Source: CAD feature listing. Evaluate the final solid. Frame: model axes, mm. A direction names the side the tool comes from. Give positions to 0.01 mm unless a question says otherwise; leave off trailing zeros. Loops run counter-clockwise (first coordinate to the right, second up) from the corner with the lowest first, then second, coordinate; pieces in that order, holes last.
```python
from build123d import *

# Parameters (mm, degrees)
F0_W     = 56.8
F0_H     = 54
F1_DEPTH = 1.8
F2_W     = 23.4
F2_H     = 12.8
F2_R     = 0.85
F3_DEPTH = 1.801
F4_R     = 1.5
F5_R     = 1.75
F5_R_2   = 0.85
F6_DEPTH = 1.4
F7_R     = 4.5
F8_DEPTH = 0.2


# Not quite as in the source:
# - a pattern or mirror of a feature is missing from the dataset's text; its kind, count and spacing are read off the source's solid


with BuildPart() as f1:
    # F0 (on Top) → F1 (new body)
    with BuildSketch(Plane.XY):
        Rectangle(F0_W, F0_H)
    extrude(amount=F1_DEPTH)

    # F2 (on face) → F3 (cut, through all)
    with BuildSketch(Plane.XY.offset(1.8)):
        with Locations((6.7, 10.6)):
            Rectangle(F2_W, F2_H)
        with Locations((-7.05, 10.6)):
            Circle(F2_R)
        with Locations((20.45, 10.6)):
            Circle(F2_R)
    f3 = extrude(amount=-F3_DEPTH, mode=Mode.SUBTRACT)

    # F3_copies: F3 across plane
    add(f3.mirror(Plane(origin=(0, 0, 0), x_dir=(0, 0, -1), z_dir=(0, -1, 0))), mode=Mode.SUBTRACT)

    # F4
    f4_edges = [f1.edges().sort_by_distance(p)[0] for p in [
        (28.4, 27, 0.9),
        (28.4, -27, 0.9),
        (-28.4, -27, 0.9),
        (-28.4, 27, 0.9),
    ]]
    fillet(f4_edges, radius=F4_R)

    # F5 (on face) → F6 (join)
    with BuildSketch(Plane(origin=(0, 0, 0), x_dir=(1, 0, 0), z_dir=(0, 0, -1))):
        with BuildLine():
            Line((-28.4, 25.5), (-28.4, -25.5))
            ThreePointArc((-28.4, -25.5), (-27.9606601718, -26.5606601718), (-26.9, -27))
            Line((-26.9, -27), (26.9, -27))
            ThreePointArc((26.9, -27), (27.9606601718, -26.5606601718), (28.4, -25.5))
            Line((28.4, -25.5), (28.4, 25.5))
            ThreePointArc((28.4, 25.5), (27.9606601718, 26.5606601718), (26.9, 27))
            Line((26.9, 27), (-26.9, 27))
            ThreePointArc((-26.9, 27), (-27.9606601718, 26.5606601718), (-28.4, 25.5))
        make_face()
        with BuildLine():
            Line((26.8, -2), (26.8, -24.4))
            ThreePointArc((26.8, -24.4), (26.5071067812, -25.1071067812), (25.8, -25.4))
            Line((25.8, -25.4), (-25.8, -25.4))
            ThreePointArc((-25.8, -25.4), (-26.5071067812, -25.1071067812), (-26.8, -24.4))
            Line((-26.8, -24.4), (-26.8, -2))
            Line((-26.8, -2), (-26.8, 2))
            Line((-26.8, 2), (-26.8, 24.4))
            ThreePointArc((-26.8, 24.4), (-26.5071067812, 25.1071067812), (-25.8, 25.4))
            Line((-25.8, 25.4), (25.8, 25.4))
            ThreePointArc((25.8, 25.4), (26.5071067812, 25.1071067812), (26.8, 24.4))
            Line((26.8, 24.4), (26.8, 2))
            Line((26.8, 2), (26.8, -2))
        make_face(mode=Mode.SUBTRACT)
        with Locations((-7.05, 10.6)):
            Circle(F5_R)
        with Locations((-7.05, 10.6)):
            Circle(F5_R_2, mode=Mode.SUBTRACT)
        with Locations((-7.05, -10.6)):
            Circle(F5_R)
        with Locations((-7.05, -10.6)):
            Circle(F5_R_2, mode=Mode.SUBTRACT)
        with Locations((20.45, 10.6)):
            Circle(F5_R)
        with Locations((20.45, 10.6)):
            Circle(F5_R_2, mode=Mode.SUBTRACT)
        with Locations((20.45, -10.6)):
            Circle(F5_R)
        with Locations((20.45, -10.6)):
            Circle(F5_R_2, mode=Mode.SUBTRACT)
        with BuildLine():
            ThreePointArc((25.6, -0.8), (26.4485281374, -1.1514718626), (26.8, -2))
            Line((26.8, -2), (26.8, 2))
            ThreePointArc((26.8, 2), (26.4485281374, 1.1514718626), (25.6, 0.8))
            Line((25.6, 0.8), (-25.6, 0.8))
            ThreePointArc((-25.6, 0.8), (-26.4485281374, 1.1514718626), (-26.8, 2))
            Line((-26.8, 2), (-26.8, -2))
            ThreePointArc((-26.8, -2), (-26.4485281374, -1.1514718626), (-25.6, -0.8))
            Line((-25.6, -0.8), (25.6, -0.8))
        make_face()
    extrude(amount=F6_DEPTH)

    # F7 (on face) → F8 (join)
    with BuildSketch(Plane.XY.offset(1.8)):
        with Locations((-26.9, 25.5)):
            Circle(F7_R)
        with Locations((-26.9, -25.5)):
            Circle(F7_R)
        with Locations((26.9, -25.5)):
            Circle(F7_R)
        with Locations((26.9, 25.5)):
            Circle(F7_R)
    extrude(amount=-F8_DEPTH)


solid = f1.part
```
(1) First-contact query: pin 1 (0.5 mm diameter, centred on x = 8, z = 1, fed in from -Y); pin 2 (1.4 mm diameter, centred on y = -12, z = 1, fed in from +X); pin 3 (0.9 mm diameter, centred on x = 1.5, z = 1, fed in from +Y). Flat tips, straight axial feed; report the tip coordinate or a pass-through.
A:
pin 1: stops at y = -27
pin 2: stops at x = 28.4
pin 3: stops at y = 27
(2) Ray query, line 1 along Y through (x, z) = (20.45, 1.1); line 2 along Y through (x, z) = (0, 1.05); line 3 along X through (y, z) = (-10.6, 0.8). Return the intervals inside material, ascending.
A:
line 1: y = -27 to -11.45, -9.75 to 9.75, 11.45 to 27
line 2: y = -27 to -17, -4.2 to 4.2, 17 to 27
line 3: x = -28.4 to -7.9, -6.2 to -5, 18.4 to 19.6, 21.3 to 28.4
(3) Section C-C, the plane z = 0.55. Return the cut outline in (x, y).
A:
outline: (-28.4, -25.5) arc R1.5 ccw to (-26.9, -27) - (26.9, -27) arc R1.5 ccw to (28.4, -25.5) - (28.4, 25.5) arc R1.5 ccw to (26.9, 27) - (-26.9, 27) arc R1.5 ccw to (-28.4, 25.5) - close; hole circle Ø1.7 at (-7.05, -10.6); hole circle Ø1.7 at (-7.05, 10.6); hole (-5, -17) - (18.4, -17) - (18.4, -4.2) - (-5, -4.2) - close; hole (-5, 4.2) - (18.4, 4.2) - (18.4, 17) - (-5, 17) - close; hole circle Ø1.7 at (20.45, -10.6); hole circle Ø1.7 at (20.45, 10.6)
(4) Section D-D, the plane y = -10.6. Return the cut outline in (x, z), then the cut area to 3 significant figures.
A:
outline: (-28.4, -1.4) - (-26.8, -1.4) - (-26.8, 0) - (-8.8, 0) - (-8.8, -1.4) - (-7.9, -1.4) - (-7.9, 1.8) - (-28.4, 1.8) - close; (-6.2, -1.4) - (-5.3, -1.4) - (-5.3, 0) - (-5, 0) - (-5, 1.8) - (-6.2, 1.8) - close; (18.4, 0) - (18.7, 0) - (18.7, -1.4) - (19.6, -1.4) - (19.6, 1.8) - (18.4, 1.8) - close; (21.3, -1.4) - (22.2, -1.4) - (22.2, 0) - (26.8, 0) - (26.8, -1.4) - (28.4, -1.4) - (28.4, 1.8) - (21.3, 1.8) - close
area: 63.5 mm2
(5) Section A-A, the plane x = 20.45. Return the cut outline in (y, z), then the cut area to 3 significant figures.
A:
outline: (-27, -1.4) - (-25.4, -1.4) - (-25.4, 0) - (-12.35, 0) - (-12.35, -1.4) - (-11.45, -1.4) - (-11.45, 1.8) - (-27, 1.8) - close; (-9.75, -1.4) - (-8.85, -1.4) - (-8.85, 0) - (-0.8, 0) - (-0.8, -1.4) - (0.8, -1.4) - (0.8, 0) - (8.85, 0) - (8.85, -1.4) - (9.75, -1.4) - (9.75, 1.8) - (-9.75, 1.8) - close; (11.45, -1.4) - (12.35, -1.4) - (12.35, 0) - (25.4, 0) - (25.4, -1.4) - (27, -1.4) - (27, 1.8) - (11.45, 1.8) - close
area: 103 mm2
(6) Section B-B, the plane y = 16. Return the cut outline in (x, z), then the cut area to 3 significant figures.
A:
outline: (-28.4, -1.4) - (-26.8, -1.4) - (-26.8, 0) - (-5, 0) - (-5, 1.8) - (-28.4, 1.8) - close; (18.4, 0) - (26.8, 0) - (26.8, -1.4) - (28.4, -1.4) - (28.4, 1.8) - (18.4, 1.8) - close
area: 64.6 mm2
(7) Reachability of faces 1 (the flat face through (0, 0, -1.4)), 2 (the cylindrical face through (-7.43, -8.89, -0.69)), 3 (the flat face through (-28, 27, 1.6)), 4 (the flat face through (-5, -11, 1)) from +Z, -Z, +X, -X, +Y, -Y: full face, straight path, thin tool, end or side. Return the list, or none.
A:
face 1: -Z, +X, -X, +Y, -Y
face 2: -Z
face 3: -Z, -X, +Y
face 4: +Z, -Z
(8) Mould query, pull axis Y, two halves, no side actions, for faces 5 (the flat face through (-28, -27, 1.6)), 6 (the cylindrical face through (-7.161, -11.443, 0.222)). Classes: pulls with the +Y half, pulls with the -Y half, needs draft (parallel to the pull), parting line crosses it, or undercut.
A:
face 5: needs draft
face 6: undercut
